Geometry check sheet. Reference: the model listing, model coordinates, mm. Face numbers are marked on the shaded views. A direction names the side the tool comes from. Give positions to 0.01 mm unless a question says otherwise; leave off trailing zeros. Loops run counter-clockwise (first coordinate to the right, second up) from the corner with the lowest first, then second, coordinate; pieces in that order, holes last.
```python
from build123d import *

# Parameters (mm, degrees)
MODEL_R                  = 18.5
MODEL_R_2                = 1.25
MODEL_R_3                = 6
RESSALTO_EXTRUS_O1_DEPTH = 21
ESBO_O2_R                = 18.25
RESSALTO_EXTRUS_O5_DEPTH = 32
ESBO_O3_R                = 6
RESSALTO_EXTRUS_O6_DEPTH = 27
ESBO_O4_R                = 2
RESSALTO_EXTRUS_O7_DEPTH = 15


with BuildPart() as part:
    # Model → Ressalto-extrusão1 (new body)
    with BuildSketch(Plane.XY):
        with Locations((7.003, 0.02)):
            Circle(MODEL_R)
        with Locations((20.777, -9.842)):
            Circle(MODEL_R_2, mode=Mode.SUBTRACT)
        with Locations((23.953, 0)):
            Circle(MODEL_R_2, mode=Mode.SUBTRACT)
        with Locations((20.777, 9.842)):
            Circle(MODEL_R_2, mode=Mode.SUBTRACT)
        with Locations((7.003, 16.95)):
            Circle(MODEL_R_2, mode=Mode.SUBTRACT)
        with Locations((-6.771, 9.842)):
            Circle(MODEL_R_2, mode=Mode.SUBTRACT)
        with Locations((-6.771, -9.842)):
            Circle(MODEL_R_2, mode=Mode.SUBTRACT)
        with Locations((7.003, -16.95)):
            Circle(MODEL_R_2, mode=Mode.SUBTRACT)
        Circle(MODEL_R_3, mode=Mode.SUBTRACT)
    extrude(amount=RESSALTO_EXTRUS_O1_DEPTH)

    # Esboço2 → Ressalto-extrusão5 (add)
    with BuildSketch(Plane.XY.offset(21)):
        with Locations((7.003, 0.02)):
            Circle(ESBO_O2_R)
    extrude(amount=RESSALTO_EXTRUS_O5_DEPTH)

    # Esboço3 → Ressalto-extrusão6 (add)
    with BuildSketch(Plane(origin=(0, 0, 21), x_dir=(-1, 0, 0), z_dir=(0, 0, -1))):
        Circle(ESBO_O3_R)
    extrude(amount=RESSALTO_EXTRUS_O6_DEPTH)

    # Esboço4 → Ressalto-extrusão7 (add)
    with BuildSketch(Plane(origin=(0, 0, -6), x_dir=(-1, 0, 0), z_dir=(0, 0, -1))):
        Circle(ESBO_O4_R)
    extrude(amount=RESSALTO_EXTRUS_O7_DEPTH)


solid = part.part
```
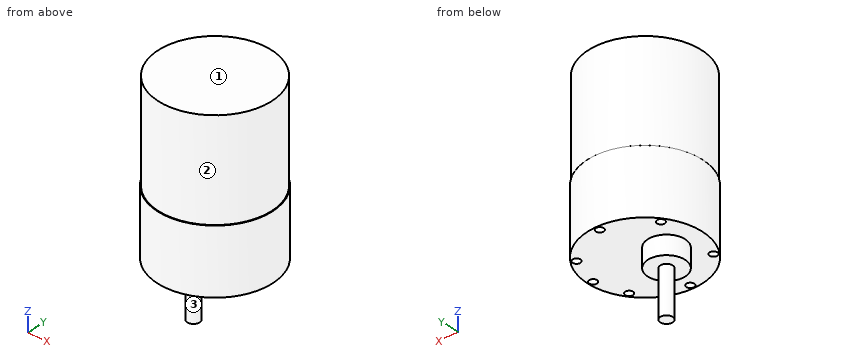
1) Sectioned sample at A-A on y = -16.95. Enter the section's corners in (x, z), plus the area to 3 significant figures.
2) Sectioned sample at D-D on z = 4.5. Enter the section's corners in (x, y), plus the area to 3 significant figures.
3) Tool access check on the marked faces 1, 2 and 3. Record the directions out of +Z, -Z, +X, -X, +Y, -Y that give a thin tool (end or side, any length) a straight path to the whole face; none if there is none.
4) Scan lines: line 1 along Z through (x, y) = (5, -2); line 2 along Z through (x, y) = (16, -16); line 3 along X through (y, z) = (12.5, 18.5). Record each from-to range of solid material in increasing order.
5) Sectioned sample at C-C on z = 46. Enter the section's corners in (x, y), plus the area to 3 significant figures.
6) Depth check by flat-ended pin: P1, Ø2, axis at x = 7.5, y = -17, coming from the -Z side; P2, Ø0.8, axis at x = -6.5, y = -10, coming from the -Z side; P3, Ø10, axis at x = -2, z = -10.5, coming from the +Y side. Enter the tip coordinate at first touch or a pass-through.
7) Sectioned sample at B-B on x = -3. Enter the section's corners in (y, z).
Determined:
1. outline: (-0.36, 0) - (5.75, 0) - (5.75, 21) - (8.25, 21) - (8.25, 0) - (14.37, 0) - (14.37, 21) - (13.72, 21) - (13.72, 53) - (0.29, 53) - (0.29, 21) - (-0.36, 21) - close
1. area: 687 mm2
2. outline: circle Ø37 at (7, 0.02); hole circle Ø2.5 at (-6.77, -9.84); hole circle Ø2.5 at (-6.77, 9.84); hole circle Ø2.5 at (7, -16.95); hole circle Ø2.5 at (7, 16.95); hole circle Ø2.5 at (20.78, -9.84); hole circle Ø2.5 at (20.78, 9.84); hole circle Ø2.5 at (23.95, 0)
2. area: 1,040 mm2
3. face 1: +Z, +X, -X, +Y, -Y
3. face 2: +Z
3. face 3: -Z
4. line 1: z = -6 to 53
4. line 2: z = 0 to 21
4. line 3: x = -6.65 to 20.66
5. outline: circle Ø36.5 at (7, 0.02)
5. area: 1,050 mm2
6. P1: stops at z = 0
6. P2: stops at z = 21
6. P3: stops at y = 6
7. outline: (-15.54, 0) - (-5.2, 0) - (-5.2, -6) - (5.2, -6) - (5.2, 0) - (15.58, 0) - (15.58, 21) - (15.28, 21) - (15.28, 53) - (-15.24, 53) - (-15.24, 21) - (-15.54, 21) - close
